Model file for the job. Use its own axes, mm. Face numbers are marked on the shaded views. Round coordinates to 2 decimals unless told otherwise and drop trailing zeros. Loops run counter-clockwise (first coordinate to the right, second up) from the corner with the lowest first, then second, coordinate; pieces in that order, holes last. Notation, with made-up numbers: (11, -12) - (44, -12) arc R26 ccw to (44, 23) - close; hole circle Ø2 at (10.25, -27.75). An arc over 180 degrees is marked (long way). Use one line per item in the form item = value.
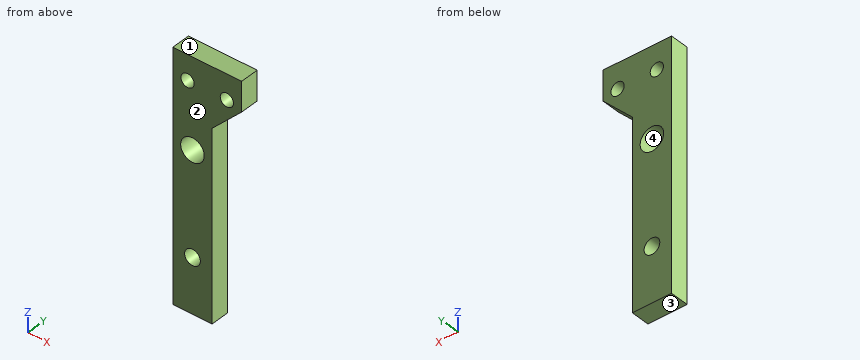
from build123d import *

# Parameters (mm, degrees)
SKETCH2_W               = 20
SKETCH2_H               = 100
SKETCH2_R               = 6
SKETCH2_R_2             = 4
BOSS_EXTRUDE1_DEPTH     = 9.525
SKETCH4_W               = 20
SKETCH4_H               = 25.4
BOSS_EXTRUDE2_DEPTH     = 9.525
BOSS_EXTRUDE3_DEPTH     = 9.525
F_1_4_CLEARANCE_HOLE2_D = 6.7564


with BuildPart() as part:
    # Sketch2 → Boss-Extrude1 (new body)
    with BuildSketch(Plane(origin=(0, 0, 0), x_dir=(1, 0, 0), z_dir=(0, 1, 0))):
        with Locations((10, -50)):
            Rectangle(SKETCH2_W, SKETCH2_H)
        with Locations(Location((10, -80, 0), (0, 0, 90))):
            Circle(SKETCH2_R, mode=Mode.SUBTRACT)
        with Locations(Location((10, -27.7, 0), (0, 0, 90))):
            Circle(SKETCH2_R_2, mode=Mode.SUBTRACT)
    extrude(amount=BOSS_EXTRUDE1_DEPTH)

    # Sketch4 → Boss-Extrude2 (add)
    with BuildSketch(Plane(origin=(0, 9.525, 0), x_dir=(1, 0, 0), z_dir=(0, 1, 0))):
        with Locations((10, -112.7)):
            Rectangle(SKETCH4_W, SKETCH4_H)
    extrude(amount=-BOSS_EXTRUDE2_DEPTH)

    # Sketch8 → Boss-Extrude3 (add)
    with BuildSketch(Plane(origin=(0, 9.525, 0), x_dir=(1, 0, 0), z_dir=(0, 1, 0))):
        Polygon((20, -125.4), (35, -125.4), (35, -110.4), (20, -95.4), align=None)
    extrude(amount=-BOSS_EXTRUDE3_DEPTH)

    # 1/4 Clearance Hole2 (through all)
    with Locations(Plane(origin=(0, 9.525, 0), x_dir=(1, 0, 0), z_dir=(0, 1, 0))):
        with Locations((7.5, -112.7), (27.5, -112.7)):
            Hole(F_1_4_CLEARANCE_HOLE2_D / 2)


solid = part.part
1. Cut at C-C, the plane x = 7.5. Give the cut face in (y, z) (1 decimal).
Geometry check:
outline = (0, 0) - (9.5, 0) - (9.5, 24.6) - (0, 24.6) - close; (0, 30.8) - (9.5, 30.8) - (9.5, 74.5) - (0, 74.5) - close; (0, 85.5) - (9.5, 85.5) - (9.5, 109.3) - (0, 109.3) - close; (0, 116.1) - (9.5, 116.1) - (9.5, 125.4) - (0, 125.4) - close
2. Flat gauge pins, fed straight in: pin 1 (6.5 mm diameter, centred on x = 10, z = 27.7, fed in from -Y); pin 2 (3 mm diameter, centred on y = 4, z = 48.5, fed in from +X). Where does each tip first touch, or does it go through?
Geometry check:
pin_1 = through
pin_2 = 20
3. Cut at D-D, the plane z = 27.7. Give the cut face in (x, y) (3 decimals).
Geometry check:
outline = (0, 0) - (6, 0) - (6, 9.525) - (0, 9.525) - close; (14, 0) - (20, 0) - (20, 9.525) - (14, 9.525) - close
4. Cut at A-A, the plane z = 112.7. Give the cut face in (x, y) (3 decimals), plus the area to 3 significant figures.
Geometry check:
outline = (0, 0) - (4.122, 0) - (4.122, 9.525) - (0, 9.525) - close; (10.878, 0) - (24.122, 0) - (24.122, 9.525) - (10.878, 9.525) - close; (30.878, 0) - (35, 0) - (35, 9.525) - (30.878, 9.525) - close
area = 205 mm^2
5. Pull direction Z, two halves, no side cores. Call the marked faces 1, 2, 3 and 4: +Z half, -Z half, draft (parallel to the pull), parting line (faces both ways), or undercut.
Geometry check:
face_1 = +Z half
face_2 = draft
face_3 = -Z half
face_4 = undercut
6. Wall check: probe 1 along X at (y, z) = (6, 112.7); probe 2 along Z at (x, y) = (12, 3); probe 3 along X at (y, z) = (7.5, 80). Give the ranges that are in metal, low to high.
Geometry check:
probe_1 = 0 to 4.12, 10.88 to 24.12, 30.88 to 35
probe_2 = 0 to 24.24, 31.16 to 74.34, 85.66 to 125.4
probe_3 = 0 to 4, 16 to 20
7. Cut at B-B, the plane y = 7.5. Give the cut face in (x, z), plus the area to 3 significant figures.
Geometry check:
outline = (0, 0) - (20, 0) - (20, 95.4) - (35, 110.4) - (35, 125.4) - (0, 125.4) - close; hole circle Ø12 at (10, 80); hole circle Ø6.76 at (7.5, 112.7); hole circle Ø8 at (10, 27.7); hole circle Ø6.76 at (27.5, 112.7)
area = 2,610 mm^2
